Can you work these out from the model? Positions are in its coordinate system, mm. A direction names the side the tool comes from. Round coordinates to 2 decimals unless told otherwise and drop trailing zeros. Loops run counter-clockwise (first coordinate to the right, second up) from the corner with the lowest first, then second, coordinate; pieces in that order, holes last. Notation, with made-up numbers: M 43,34.25 L 88,34.25 A26 ccw 88,62.25 Z; hole C 2,66.5 d11. An arc over 180 degrees is marked long. Answer as CSV lines item,"result".
from build123d import *

# Parameters (mm, degrees)
F0_R     = 14.2875
F0_R_2   = 15.875
F0_R_3   = 3.175
F1_DEPTH = 4.7625


with BuildPart() as f1:
    # F0 (on Front) → F1 (new body)
    with BuildSketch(Plane.XZ):
        with BuildLine():
            ThreePointArc((320.379174, 54.839155), (328.771893, 68.117601), (331.705949, 83.549587))
            Line((331.705949, 83.549587), (331.705949, 114.540323))
            ThreePointArc((331.705949, 114.540323), (329.846077, 119.030451), (325.355949, 120.890323))
            Line((325.355949, 120.890323), (0, 120.890323))
            Line((0, 120.890323), (-325.355949, 120.890323))
            ThreePointArc((-325.355949, 120.890323), (-329.846077, 119.030451), (-331.705949, 114.540323))
            Line((-331.705949, 114.540323), (-331.705949, 83.549587))
            ThreePointArc((-331.705949, 83.549587), (-328.771893, 68.117601), (-320.379174, 54.839155))
            ThreePointArc((-320.379174, 54.839155), (-309.670458, 47.826041), (-296.934801, 46.536319))
            ThreePointArc((-296.934801, 46.536319), (-269.099557, 42.644178), (-247.49135, 24.671004))
            ThreePointArc((-247.49135, 24.671004), (-235.295113, 14.866395), (-219.708208, 13.478246))
            ThreePointArc((-219.708208, 13.478246), (-186.874924, 11.834063), (-159.034985, -5.649233))
            ThreePointArc((-159.034985, -5.649233), (-144.789086, -13.599949), (-128.564673, -11.888835))
            ThreePointArc((-128.564673, -11.888835), (-67.876372, 4.053452), (-5.219212, 0.690928))
            ThreePointArc((-5.219212, 0.690928), (-2.623901, 0.279775), (0, 0.138953))
            ThreePointArc((0, 0.138953), (2.623901, 0.279775), (5.219212, 0.690928))
            ThreePointArc((5.219212, 0.690928), (36.620267, 4.819782), (68.281297, 4.011744))
            ThreePointArc((68.281297, 4.011744), (99.037359, -1.609285), (128.564673, -11.888835))
            ThreePointArc((128.564673, -11.888835), (144.789086, -13.599949), (159.034985, -5.649233))
            ThreePointArc((159.034985, -5.649233), (171.832729, 4.879417), (186.874924, 11.834063))
            ThreePointArc((186.874924, 11.834063), (203.186029, 14.763672), (219.708208, 13.478246))
            ThreePointArc((219.708208, 13.478246), (235.295113, 14.866395), (247.49135, 24.671004))
            ThreePointArc((247.49135, 24.671004), (269.099557, 42.644178), (296.934801, 46.536319))
            ThreePointArc((296.934801, 46.536319), (309.670458, 47.826041), (320.379174, 54.839155))
        make_face()
        with Locations((-139.375032, 12.838909)):
            Circle(F0_R, mode=Mode.SUBTRACT)
        with Locations((-225.210487, 39.898884)):
            Circle(F0_R, mode=Mode.SUBTRACT)
        with Locations((-0.047461, 25.538909)):
            Circle(F0_R_2, mode=Mode.SUBTRACT)
        with Locations((139.375032, 12.838909)):
            Circle(F0_R, mode=Mode.SUBTRACT)
        with Locations((225.210487, 39.898884)):
            Circle(F0_R, mode=Mode.SUBTRACT)
        with Locations((-300.661124, 73.265323)):
            Circle(F0_R, mode=Mode.SUBTRACT)
        with Locations((-224.775985, 112.751594)):
            Circle(F0_R_3, mode=Mode.SUBTRACT)
        with Locations((-173.975985, 112.751594)):
            Circle(F0_R_3, mode=Mode.SUBTRACT)
        with Locations((-25.4, 112.751594)):
            Circle(F0_R_3, mode=Mode.SUBTRACT)
        with Locations((300.661124, 73.265323)):
            Circle(F0_R, mode=Mode.SUBTRACT)
        with Locations((25.4, 112.751594)):
            Circle(F0_R_3, mode=Mode.SUBTRACT)
        with Locations((166.605949, 112.751594)):
            Circle(F0_R_3, mode=Mode.SUBTRACT)
        with Locations((217.405949, 112.751594)):
            Circle(F0_R_3, mode=Mode.SUBTRACT)
    extrude(amount=F1_DEPTH)


solid = f1.part
Item 1: On a 3-axis mill with a long thin cutter (end or side, diameter ignored), from which of +Z, -Z, +X, -X, +Y, -Y can I reach the whole of each face in a straight line? I mean faces 4 (the face through (98.614, -2.348, -1.498)), 5 (the face through (171.64, -2.35, 4.76)). Say none if no direction works.
Output:
face 4,"-Z, +Y, -Y"
face 5,"-Z, +X, +Y, -Y"
Item 2: If we section it at A-A on x = 232: Write out the boundary of the cut face in (y, z), then the cut area to 3 significant figures.
Output:
outline,"M -4.76,13.78 L 0,13.78 L 0,27.33 L -4.76,27.33 Z; M -4.76,52.47 L 0,52.47 L 0,120.89 L -4.76,120.89 Z"
area,"390 mm2"
Item 3: If we section it at D-D on x = 85: Write out the boundary of the cut face in (y, z), then the cut area to 3 significant figures.
Output:
outline,"M -4.76,1.57 L 0,1.57 L 0,120.89 L -4.76,120.89 Z"
area,"568 mm2"
Item 4: Will these pins go through, and if not, where does the flat tip stop? pin 1 (10 mm diameter, centred on x = 236.5, z = 8.5, fed in from -Y); pin 2 (1 mm diameter, centred on y = -3, z = 30, fed in from -X); pin 3 (1.5 mm diameter, centred on y = -0.5, z = 80, fed in from -X).
Output:
pin 1,"passes through"
pin 2,"stops at x = -252.13"
pin 3,"stops at x = -331.61"
Item 5: If we section it at C-C on y = -3.85: State how many separate pieces and enclosed holes the cut face has, then the cut area to 3 significant figures.
Output:
separate pieces,"1"
enclosed holes,"13"
area,"66,000 mm2"
Item 6: We'd pull the mould along X, two halves only. Please class faces 1 (the face through (-287.463, -2.348, 67.793)), 2 (the face through (-5, 0, 69)), 3 (the face through (328.69, -2.35, 67.91)): released by +X, released by -X, zero draft, split by the parting line, or undercut.
Output:
face 1,"undercut"
face 2,"zero draft"
face 3,"released by +X"
Item 7: If we section it at B-B on z = 33: Write out the boundary of the cut face in (x, y).
Output:
outline,"M -254.6,-4.76 L -237.72,-4.76 L -237.72,0 L -254.6,0 Z; M -212.7,-4.76 L -14.06,-4.76 L -14.06,0 L -212.7,0 Z; M 13.96,-4.76 L 212.7,-4.76 L 212.7,0 L 13.96,0 Z; M 237.72,-4.76 L 254.6,-4.76 L 254.6,0 L 237.72,0 Z"
Item 8: If I drill on line 1 along X through (y, z) = (-2.55, 66.5); line 2 along X through (y, z) = (-4.4, 85); line 3 along X through (y, z) = (-1, 29.5), over which ranges is the centre line in solid material (lowest first)? Write a range as from..to.
Output:
line 1,"x = -328.09..-313.25, -288.08..288.08, 313.25..328.09"
line 2,"x = -331.71..-308.81, -292.51..292.51, 308.81..331.71"
line 3,"x = -251.23..-235.01, -215.41..-15.42, 15.33..215.41, 235.01..251.23"
